```python
from build123d import *

# Parameters (mm, degrees)
SKETCH1_R           = 11
SKETCH1_R_2         = 1.5
SKETCH1_W           = 5
SKETCH1_H           = 6
BOSS_EXTRUDE1_DEPTH = 5


with BuildPart() as part:
    # Sketch1 → Boss-Extrude1 (new body)
    with BuildSketch(Plane(origin=(0, 0, 0), x_dir=(1, 0, 0), z_dir=(0, 1, 0))):
        with BuildLine():
            Line((40.393958783, 14.993950885), (40.393958783, -25.006049115))
            ThreePointArc((40.393958783, -25.006049115), (41.862698298, -28.539809641), (45.4, -30))
            Line((45.4, -30), (54.2, -30))
            Line((54.2, -30), (54.2, -55))
            Line((54.2, -55), (41.099999997, -55))
            Line((41.099999997, -55), (41.099999997, -63))
            Line((41.099999997, -63), (-23.900000003, -63))
            Line((-23.900000003, -63), (-23.900000003, -55))
            Line((-23.900000003, -55), (-37.00036842, -55))
            ThreePointArc((-37.00036842, -55), (-42.656802211, -52.657122122), (-45.000000024, -47.000820858))
            Line((-45.000000024, -47.000820858), (-45.000000024, 15.001139744))
            ThreePointArc((-45.000000024, 15.001139744), (-36.213537283, 36.213537259), (-15.001139768, 45))
            Line((-15.001139768, 45), (10.397234849, 44.997226593))
            ThreePointArc((10.397234849, 44.997226593), (31.609478673, 36.208113679), (40.393958783, 14.993950885))
        make_face()
        Circle(SKETCH1_R, mode=Mode.SUBTRACT)
        with Locations((9.89288341, 9.906102051)):
            Circle(SKETCH1_R_2, mode=Mode.SUBTRACT)
        with Locations((9.89288341, -9.906102051)):
            Circle(SKETCH1_R_2, mode=Mode.SUBTRACT)
        with Locations((-9.89288341, -9.906102051)):
            Circle(SKETCH1_R_2, mode=Mode.SUBTRACT)
        with Locations((-9.89288341, 9.906102051)):
            Circle(SKETCH1_R_2, mode=Mode.SUBTRACT)
        with Locations((-9.400000003, -59)):
            Circle(SKETCH1_R_2, mode=Mode.SUBTRACT)
        with Locations((26.599999997, -59)):
            Circle(SKETCH1_R_2, mode=Mode.SUBTRACT)
        with Locations((-30.000000024, -40)):
            Circle(SKETCH1_R_2, mode=Mode.SUBTRACT)
        with Locations((36.599999976, -40)):
            Circle(SKETCH1_R_2, mode=Mode.SUBTRACT)
        with Locations((-39.500000024, -31)):
            Rectangle(SKETCH1_W, SKETCH1_H, mode=Mode.SUBTRACT)
        with Locations((-39.500000024, -47)):
            Rectangle(SKETCH1_W, SKETCH1_H, mode=Mode.SUBTRACT)
        with Locations((48.7, -36)):
            Rectangle(SKETCH1_W, SKETCH1_H, mode=Mode.SUBTRACT)
        with Locations((48.7, -49)):
            Rectangle(SKETCH1_W, SKETCH1_H, mode=Mode.SUBTRACT)
    extrude(amount=BOSS_EXTRUDE1_DEPTH)


solid = part.part
```
Model file for the job. Use its own axes, mm. A direction names the side the tool comes from. Coordinates: 2 decimals unless noted, no trailing zeros. Loops run counter-clockwise (first coordinate to the right, second up) from the corner with the lowest first, then second, coordinate; pieces in that order, holes last. Notation, with made-up numbers: (12.5, 38.25) - (63.5, 38.25) arc R22 ccw to (63.5, 58.25) - close; hole circle Ø7 at (88.25, 52). An arc over 180 degrees is marked (long way). Answer as a JSON object with one key per item and string values. Group by question number.
(1) Cut at A-A (z = 59). Give the cut face in (x, y), then the cut area to 3 significant figures.
(2) Probe line 1 along X through (y, z) = (1.45, 59); line 2 along X through (y, z) = (1, 40); line 3 along Z through (x, y) = (0, 1.6). List the from-to ranges inside material, lowest first.
(3) Cut at C-C (x = 0). Give the cut face in (y, z), then the cut area to 3 significant figures.
(4) Cut at B-B (x = 36.6). Give the cut face in (y, z), then the cut area to 3 significant figures.
(5) Flat gauge pins, fed straight in: pin 1 (1.5 mm diameter, centred on x = -38.5, y = 1.5, fed in from -Z); pin 2 (2 mm diameter, centred on y = 2.5, z = 28.5, fed in from +X); pin 3 (1.5 mm diameter, centred on x = -38.5, y = 2, fed in from +Z). Where does each tip first touch, or does it go through?
(6) Cut at D-D (y = 1.95). State how many separate pieces and enclosed holes the cut face has, then the cut area to 3 significant figures.
(7) Two-plate mould, pull along Z, no slides. Class faces 1 (the face through (-36.445, 2.465, -35.979)), 2 (the face through (-45, 2, 16)), 3 (the face through (9, 2, 63)), 4 (the face through (-37, 2, 31)): released by +Z, released by -Z, zero draft, split by the parting line, or undercut.
(8) Tool access for faces 5 (the face through (-40, 2, 50)), 6 (the face through (-42.594, 2.465, 52.719)), 7 (the face through (48, 2, 55)): list every direction of +Z, -Z, +X, -X, +Y, -Y with a clear straight run to the whole face (end or side of a thin tool).
Geometry says:
{
 "1": {"outline": "(-23.9, 0) - (-10.9, 0) - (-10.9, 5) - (-23.9, 5) - close; (-7.9, 0) - (25.1, 0) - (25.1, 5) - (-7.9, 5) - close; (28.1, 0) - (41.1, 0) - (41.1, 5) - (28.1, 5) - close", "area": "295 mm^2"},
 "2": {"line 1": "x = -23.9 to -10.9, -7.9 to 25.1, 28.1 to 41.1", "line 2": "x = -45 to -31.5, -28.5 to 35.1, 38.1 to 54.2", "line 3": "z = -45 to -11, 11 to 63"},
 "3": {"outline": "(0, -45) - (5, -45) - (5, -11) - (0, -11) - close; (0, 11) - (5, 11) - (5, 63) - (0, 63) - close", "area": "430 mm^2"},
 "4": {"outline": "(0, -29.6) - (5, -29.6) - (5, 38.5) - (0, 38.5) - close; (0, 41.5) - (5, 41.5) - (5, 63) - (0, 63) - close", "area": "448 mm^2"},
 "5": {"pin 1": "stops at z = -34.56", "pin 2": "stops at x = 43.21", "pin 3": "stops at z = 54.96"},
 "6": {"separate pieces": "1", "enclosed holes": "13", "area": "8,450 mm^2"},
 "7": {"face 1": "released by -Z", "face 2": "zero draft", "face 3": "released by +Z", "face 4": "undercut"},
 "8": {"face 5": "+Y, -Y", "face 6": "+Z, -X, +Y, -Y", "face 7": "+Z, +X, +Y, -Y"}
}
